Autodesk Fusion 360 part; units mm, degrees
sketch "Sketch5" plane through (0, 0, 0) normal (0, 0, 1) x (1, 0, 0)
  line L0 (0, 0) -> (225, 0)
  line L1 (225, 0) -> (225, -125)
  line L2 (225, -125) -> (0, -125)
  line L3 (0, -125) -> (0, 0)
  dimension "d26" = 225
  dimension "d27" = 125
extrude "Extrude3" add sketch "Sketch5" along normal blind 15
sketch "Sketch6" plane through (0, 0, 15) normal (0, 0, 1) x (-1, 0, 0)
  line L0 (0, 125) -> (-225, 125)
  line L1 (-225, 125) -> (-225, 0)
  line L2 (-225, 0) -> (0, 0)
  line L3 (0, 0) -> (0, 125)
  line L4 (0, 0) -> (0, 62.5) construction
  line L5 (0, 62.5) -> (-225, 62.5) construction
  line L6 (0, 62.5) -> (0, 52.5)
  line L7 (0, 62.5) -> (0, 72.5)
  line L8 (0, 52.5) -> (-225, 52.5)
  line L9 (-225, 52.5) -> (-225, 72.5)
  line L10 (-225, 72.5) -> (0, 72.5)
  dimension "d30" = 62.5
  dimension "d31" = 10
  dimension "d32" = 10
  dimension "d33" = 225
  dimension "d34" = 20
extrude "Extrude4" add sketch "Sketch6" along normal blind 100 contours L1 L3 L6 L7 L8 L9 L10
sketch "Sketch7" plane through (0, -72.5, 0) normal (0, -1, 0) x (1, 0, 0)
  line L0 (0, 15) -> (225, 15)
  line L1 (225, 15) -> (225, 115)
  line L2 (225, 115) -> (0, 115)
  line L3 (0, 115) -> (0, 15)
  line L4 (0, 15) -> (72.5, 15) construction
  arc A0 (152.5, 15) -> (72.5, 15) centre (112.5, 15) ccw
  line L5 (0, 115) -> (25, 115)
  line L6 (25, 115) -> (50, 115)
  line L7 (50, 115) -> (75, 115)
  line L8 (75, 115) -> (100, 115)
  line L9 (100, 115) -> (125, 115)
  line L10 (125, 115) -> (150, 115)
  line L11 (150, 115) -> (175, 115)
  line L12 (175, 115) -> (200, 115)
  line L13 (200, 115) -> (225, 115)
  circle A1 centre (12.5, 115) radius 7.5
  circle A2 centre (62.5, 115) radius 7.5
  circle A3 centre (112.5, 115) radius 7.5
  circle A4 centre (162.5, 115) radius 7.5
  circle A5 centre (212.5, 115) radius 7.5
  line L14 (25, 115) -> (25, 95)
  line L15 (25, 95) -> (50, 95)
  line L16 (50, 95) -> (50, 115)
  line L17 (75, 115) -> (75, 95)
  line L18 (75, 95) -> (100, 95)
  line L19 (100, 95) -> (100, 115)
  line L20 (125, 115) -> (125, 95)
  line L21 (125, 95) -> (150, 95)
  line L22 (150, 95) -> (150, 115)
  line L23 (175, 115) -> (175, 95)
  line L24 (175, 95) -> (200, 95)
  line L25 (200, 95) -> (200, 115)
  arc A6 (25, 115) -> (0, 115) centre (12.5, 115) ccw
  arc A7 (75, 115) -> (50, 115) centre (62.5, 115) ccw
  arc A8 (125, 115) -> (100, 115) centre (112.5, 115) ccw
  arc A9 (175, 115) -> (150, 115) centre (162.5, 115) ccw
  arc A10 (225, 115) -> (200, 115) centre (212.5, 115) ccw
  point P0 (62.5, 115)
  point P1 (112.5, 115)
  point P2 (162.5, 115)
  point P3 (212.5, 115)
  dimension "d37" = 112.5
  dimension "d38" = 80
  dimension "d42" = 25
  dimension "d43" = 25
  dimension "d44" = 25
  dimension "d45" = 25
  dimension "d46" = 25
  dimension "d47" = 25
  dimension "d48" = 25
  dimension "d49" = 25
  dimension "d50" = 25
  dimension "d51" = 15
  dimension "d52" = 25
  dimension "d55" = 200
  dimension "d56" = 0
  dimension "d57" = 20
  dimension "d62" = 100
extrude "Extrude5" cut sketch "Sketch7" against normal blind 20 contours L0 A0
extrude "Extrude6" add sketch "Sketch7" against normal blind 20 contours L2 L5 A1 A6 | L2 L5 A1 | L2 L5 A1 | L2 L7 A2 A7 | L2 L13 A5 A10 | L2 L7 A2 | L2 L13 A5 | L2 L9 A3 A8 | L2 L11 A4 A9 | L2 L9 A3 | L2 L11 A4 picked at (63.3854, 117.6998) picked at (214.3326, 116.7004) picked at (113.3854, 117.6998) picked at (164.3326, 116.7004)
extrude "Extrude7" cut sketch "Sketch7" against normal blind 20 contours L2 L6 L14 L15 L16 | L2 L8 L17 L18 L19 | L2 L12 L23 L24 L25 | L2 L10 L20 L21 L22
extrude "Extrude8" cut sketch "Sketch7" against normal blind 20 contours L2 L5 A1 | L2 L5 A1 | L2 L7 A2 | L2 L7 A2 | L2 L13 A5 | L2 L13 A5 | L2 L9 A3 | L2 L9 A3 | L2 L11 A4 | L2 L11 A4
Part model, mm, in its own coordinate system. A direction names the side the tool comes from. Round coordinates to 2 decimals unless told otherwise and drop trailing zeros. Write each loop counter-clockwise with the first axis right and the second up, starting at its lowest first coordinate (ties: lowest second). Pieces come first, ordered by that corner, then holes. Notation, with made-up numbers: M -37,18.25 L 12,18.25 A20 ccw 12,47.25 Z; hole C -37.75,40 d7. An arc over 180 degrees is marked long. Answer as CSV lines item,"result". Start each with the question number.
1) Band-saw the part on C-C (x = 182). List the corners of the cut face in (y, z), then the cut area to 4 significant figures.
2) Which spindle directions (+Z, -Z, +X, -X, +Y, -Y) get a long thin tool onto all of the face, cutting with end or side? Do faces 1 (the face through (114, -72.5, 58)), 2 (the face through (113.38, -62.64, 54.99)), 3 (the face through (100, -63, 105)). Say none if no direction does.
3) Band-saw the part on A-A (y = -70). List the corners of the cut face in (x, z).
4) Mould opens along Z. For faces 4 (the face through (87, -63, 95)), 5 (the face through (225, -58, 36)), 6 (the face through (169.43, -62.64, 112.13)) say: +Z half, -Z half, draft (parallel to the pull), parting line (faces both ways), or undercut.
5) Band-saw the part on B-B (x = 12.5). List the corners of the cut face in (y, z).
6) Drill centre lines: L1, parallel to Z at x = 162, y = -63; L2, parallel to Y at x = 66.5, z = 74.5; L3, parallel to Z at x = 58.5, y = -23. Where is each one in solid material? Low to high.
7) Band-saw the part on D-D (z = 87). List the corners of the cut face in (x, y), then the cut area to 3 significant figures.
8) Drop flat-ended pins along their axis: pin 1 (8 mm diameter, centred on x = 184.5, y = -58.5, fed in from -Z); pin 2 (12 mm diameter, centred on x = 83, z = 56.5, fed in from -Y); pin 3 (10 mm diameter, centred on x = 167, z = 31, fed in from +Y); pin 4 (16 mm diameter, centred on x = 89.5, y = -62, fed in from +Z). Give the stop position or say it passes through.
Worked out:
1,outline,"M -125,0 L 0,0 L 0,15 L -52.5,15 L -52.5,95 L -72.5,95 L -72.5,15 L -125,15 Z"
1,area,"3,475 mm²"
2,face 1,"+Z, +X, -X, -Y"
2,face 2,"+Y, -Y"
2,face 3,"+Z, +Y, -Y"
3,outline,"M 0,0 L 225,0 L 225,115 A12.5 ccw 200,115 L 200,95 L 175,95 L 175,115 A12.5 ccw 150,115 L 150,95 L 125,95 L 125,115 A12.5 ccw 100,115 L 100,95 L 75,95 L 75,115 A12.5 ccw 50,115 L 50,95 L 25,95 L 25,115 A12.5 ccw 0,115 Z; hole C 12.5,115 d15; hole C 62.5,115 d15; hole M 72.5,15 L 152.5,15 A40 ccw Z; hole C 112.5,115 d15; hole C 162.5,115 d15; hole C 212.5,115 d15"
4,face 4,"+Z half"
4,face 5,"draft"
4,face 6,"undercut"
5,outline,"M -125,0 L 0,0 L 0,15 L -52.5,15 L -52.5,107.5 L -72.5,107.5 L -72.5,15 L -125,15 Z; M -72.5,122.5 L -52.5,122.5 L -52.5,127.5 L -72.5,127.5 Z"
6,L1,"0 to 107.52, 122.48 to 127.49"
6,L2,"-72.5 to -52.5"
6,L3,"0 to 15"
7,outline,"M 0,-72.5 L 225,-72.5 L 225,-52.5 L 0,-52.5 Z"
7,area,"4,500 mm²"
8,pin 1,"z = 0"
8,pin 2,"y = -72.5"
8,pin 3,"y = -52.5"
8,pin 4,"z = 95"
